Could you check a few things on this model? Use its own coordinates, in mm. Face numbers are marked on the shaded views. Give positions to 0.01 mm unless a question says otherwise; leave off trailing zeros. Write each loop counter-clockwise with the first axis right and the second up, starting at its lowest first coordinate (ties: lowest second). Pieces come first, ordered by that corner, then holes. Notation, with made-up numbers: (15, -14) - (70, -14) arc R23 ccw to (70, 5) - close; hole circle Ø1 at (-21.75, 5.5). An arc over 180 degrees is marked (long way). Write item = value, one per line.
from build123d import *

# Parameters (mm, degrees)
SKETCH1_W           = 16
SKETCH1_H           = 2.5
SKETCH1_W_2         = 4.041280146
SKETCH1_H_2         = 1.13793654
SKETCH1_H_3         = 1.137936541
BOSS_EXTRUDE1_DEPTH = 2.2


with BuildPart() as part:
    # Sketch1 → Boss-Extrude1 (new body)
    with BuildSketch(Plane(origin=(0, 0, 0), x_dir=(1, 0, 0), z_dir=(0, 1, 0))):
        Polygon((-135.695425431, -45.865904239), (-137.195425431, -45.865904239), (-137.195425431, -51.865904239), (-135.695425431, -51.865904239), (-135.695425431, -58.865904239), (-112.695425431, -58.865904239), (-112.695425431, -38.865904239), (-135.695425431, -38.865904239), align=None)
        with Locations((-124.945425431, -54.615904239)):
            Rectangle(SKETCH1_W, SKETCH1_H, mode=Mode.SUBTRACT)
        with Locations((-125.060873132, -50.934872509)):
            Rectangle(SKETCH1_W_2, SKETCH1_H_2, mode=Mode.SUBTRACT)
        with Locations((-125.060873132, -46.796935969)):
            Rectangle(SKETCH1_W_2, SKETCH1_H_3, mode=Mode.SUBTRACT)
        with Locations((-124.945425431, -43.115904239)):
            Rectangle(SKETCH1_W, SKETCH1_H, mode=Mode.SUBTRACT)
    extrude(amount=BOSS_EXTRUDE1_DEPTH)


solid = part.part
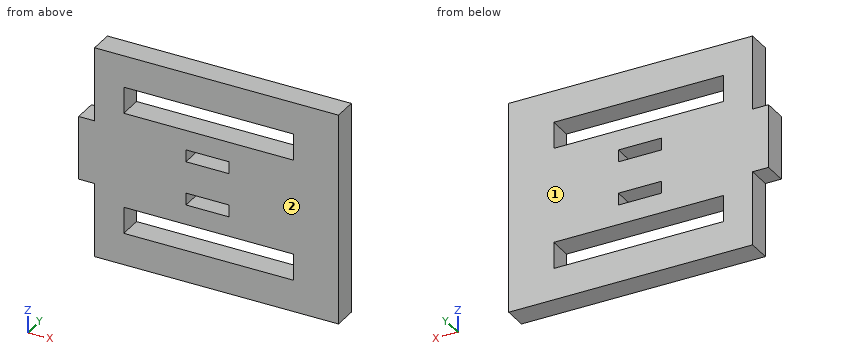
1. If we section it at D-D, the plane z = 46.5: Please give me the cut outline in (x, y), and give its area (3 significant figures).
Filled sheet:
outline = (-137.2, 0) - (-127.08, 0) - (-127.08, 2.2) - (-137.2, 2.2) - close; (-123.04, 0) - (-112.7, 0) - (-112.7, 2.2) - (-123.04, 2.2) - close
area = 45.0 mm2
2. Thinking about a two-plate mould opening in Y: for the marked faces 1 and 2, which applies, pulls with the +Y half, pulls with the -Y half, needs draft (parallel to the pull), parting line crosses it, or undercut?
Filled sheet:
face_1 = pulls with the +Y half
face_2 = pulls with the -Y half
3. For pin 1 (0.7 mm diameter, centred on y = 1, z = 55.5, fed in from -X); pin 2 (0.8 mm diameter, centred on x = -136.5, y = 0.5, fed in from +Z), each with a flat end and sliding along its axis, tell me the tip position at first contact or that it passes through.
Filled sheet:
pin_1 = -135.7
pin_2 = 51.87
4. If we section it at A-A, the plane z = 42.5: Please give me the cut outline in (x, y).
Filled sheet:
outline = (-135.7, 0) - (-132.95, 0) - (-132.95, 2.2) - (-135.7, 2.2) - close; (-116.95, 0) - (-112.7, 0) - (-112.7, 2.2) - (-116.95, 2.2) - close
5. If we section it at B-B, the plane x = -132: Please give me the cut outline in (y, z), and give its area (3 significant figures).
Filled sheet:
outline = (0, 38.87) - (2.2, 38.87) - (2.2, 41.87) - (0, 41.87) - close; (0, 44.37) - (2.2, 44.37) - (2.2, 53.37) - (0, 53.37) - close; (0, 55.87) - (2.2, 55.87) - (2.2, 58.87) - (0, 58.87) - close
area = 33.0 mm2
6. If we section it at C-C, the plane y = 0.75: Please give me the cut outline in (x, z).
Filled sheet:
outline = (-137.2, 45.87) - (-135.7, 45.87) - (-135.7, 38.87) - (-112.7, 38.87) - (-112.7, 58.87) - (-135.7, 58.87) - (-135.7, 51.87) - (-137.2, 51.87) - close; hole (-132.95, 41.87) - (-116.95, 41.87) - (-116.95, 44.37) - (-132.95, 44.37) - close; hole (-132.95, 53.37) - (-116.95, 53.37) - (-116.95, 55.87) - (-132.95, 55.87) - close; hole (-127.08, 46.23) - (-123.04, 46.23) - (-123.04, 47.37) - (-127.08, 47.37) - close; hole (-127.08, 50.37) - (-123.04, 50.37) - (-123.04, 51.5) - (-127.08, 51.5) - close
7. I need wall thicknesses on line 1 (Z direction, x = -122.25, y = 1.45); line 2 (Z direction, x = -126.75, y = 2); line 3 (X direction, y = 0.5, z = 54). Which ranges of each line are inside material? Lowest first, please.
Filled sheet:
line_1 = 38.87 to 41.87, 44.37 to 53.37, 55.87 to 58.87
line_2 = 38.87 to 41.87, 44.37 to 46.23, 47.37 to 50.37, 51.5 to 53.37, 55.87 to 58.87
line_3 = -135.7 to -132.95, -116.95 to -112.7
